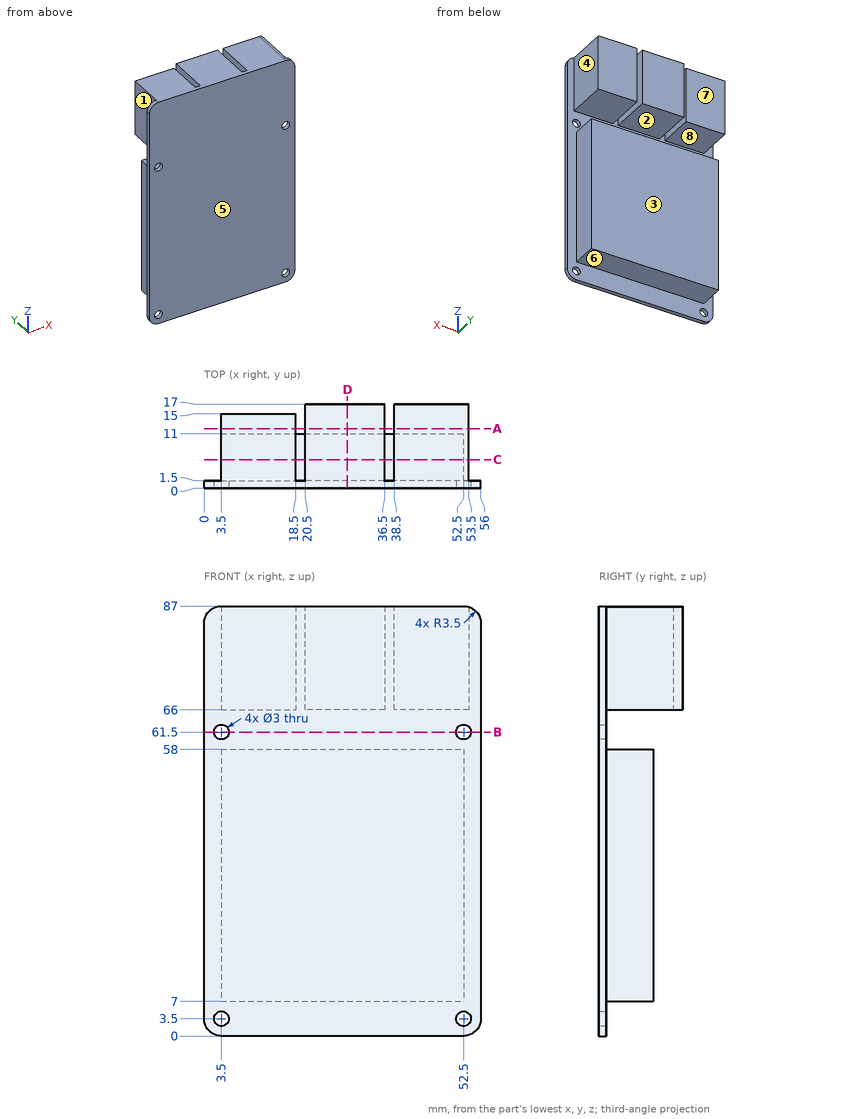
The drawing under review shows one solid part. Ordinate dimensions are in mm from its lowest x, y, z. A direction names the side the tool comes from. Round coordinates to 2 decimals unless told otherwise and drop trailing zeros. Loops run counter-clockwise (first coordinate to the right, second up) from the corner with the lowest first, then second, coordinate; pieces in that order, holes last. Notation, with made-up numbers: (89.5, 76) - (102.5, 76) arc R16 ccw to (102.5, 101) - close; hole circle Ø11 at (-12, 38.5). An arc over 180 degrees is marked (long way). Use a Markdown table: item, result. Add a question column.
Q1. Add section D-D (x = 29). State the section outline as (y, z) points.
Q2. Machinability: for the marked faces 1, 2, 3, 4 and 5, which of the approach directions +Z, -Z, +X, -X, +Y, -Y give a long, thin tool a straight path to every point of the face, cutting with its end or side? Answer none if there is none.
Q3. Add section A-A (y = 12). State the section outline as (x, z) points.
Q4. Insertion check: pin 1 Ø4.5 at (y, z) = (7, 72) entering from +X; pin 2 Ø17 at (x, z) = (32, 53) entering from +Y; pin 3 Ø5 at (y, z) = (6.5, 24.5) entering from +X. Each pin has a flat end and moves straight along its axis. Give the tip position at first contact, or say it passes through.
Q5. Add section B-B (z = 61.5). State the section outline as (x, y) points, plus the area to 3 significant figures.
Q6. Add section C-C (y = 5.75). State the section outline as (x, z) points.
Q7. For probe 1 along X at (y, z) = (0.8, 61.5); probe 2 along X at (y, z) = (2.5, 70); probe 3 along Z at (x, y) = (25, 5.75), list the stretches that pass through material, from the lowest coordinate up.
Q8. The part is to be moulded in two halves that separate along Z. For the marked faces 6, 7 and 8, say which applies: pulls with the +Z half, pulls with the -Z half, needs draft (parallel to the pull), parting line crosses it, or undercut.
Worked answers:
| question | item | result |
|---|---|---|
| 1 | outline | (0, 0) - (1.5, 0) - (1.5, 7) - (11, 7) - (11, 58) - (1.5, 58) - (1.5, 66) - (17, 66) - (17, 87) - (0, 87) - close |
| 2 | face 1 | +Z, -Z, -X, +Y |
| 2 | face 2 | +X, -X, +Y |
| 2 | face 3 | -Z, +X, -X, +Y |
| 2 | face 4 | +Z, -Z, +X, +Y |
| 2 | face 5 | +Z, -Z, +X, -X, -Y |
| 3 | outline | (3.5, 66) - (18.5, 66) - (18.5, 87) - (3.5, 87) - close; (20.5, 66) - (36.5, 66) - (36.5, 87) - (20.5, 87) - close; (38.5, 66) - (53.5, 66) - (53.5, 86.85) arc R3.5 ccw to (52.5, 87) - (38.5, 87) - close |
| 4 | pin 1 | x = 53.5 |
| 4 | pin 2 | y = 11 |
| 4 | pin 3 | x = 52.5 |
| 5 | outline | (0, 0) - (2, 0) - (2, 1.5) - (0, 1.5) - close; (5, 0) - (51, 0) - (51, 1.5) - (5, 1.5) - close; (54, 0) - (56, 0) - (56, 1.5) - (54, 1.5) - close |
| 5 | area | 75.0 mm² |
| 6 | outline | (3.5, 7) - (52.5, 7) - (52.5, 58) - (3.5, 58) - close; (3.5, 66) - (18.5, 66) - (18.5, 87) - (3.5, 87) - close; (20.5, 66) - (36.5, 66) - (36.5, 87) - (20.5, 87) - close; (38.5, 66) - (53.5, 66) - (53.5, 86.85) arc R3.5 ccw to (52.5, 87) - (38.5, 87) - close |
| 7 | probe 1 | 0 to 2, 5 to 51, 54 to 56 |
| 7 | probe 2 | 3.5 to 18.5, 20.5 to 36.5, 38.5 to 53.5 |
| 7 | probe 3 | 7 to 58, 66 to 87 |
| 8 | face 6 | pulls with the -Z half |
| 8 | face 7 | needs draft |
| 8 | face 8 | undercut |
